from build123d import *

# Parameters (mm, degrees)
EXTRUDE_1_DEPTH          = 4
FILLET_1_R               = 10
SKETCH_2_R               = 7.5
SKETCH_2_R_2             = 1.25
CUT_EXTRUDE_1_DEPTH      = 5
PATTERN_CIRCULAR_1_COUNT = 6
SKETCH_3_R               = 12.5
SKETCH_3_R_2             = 1.25
CUT_EXTRUDE_2_DEPTH      = 5
PATTERN_CIRCULAR_2_COUNT = 4
SKETCH_4_W               = 120
SKETCH_4_H               = 12
CUT_EXTRUDE_3_DEPTH      = 5
FILLET_2_R               = 6
FILLET_3_R               = 6
SKETCH_5_R               = 1.25
CUT_EXTRUDE_5_DEPTH      = 5
PATTERN_LINEAR_2_COUNT   = 3
PATTERN_LINEAR_2_PITCH   = 45


with BuildPart() as part:
    # 草图1 → 凸台-拉伸1 (new body)
    with BuildSketch(Plane.XY):
        with BuildLine():
            Line((18.319446876, 21.832266629), (161.680553124, 21.832266629))
            ThreePointArc((161.680553124, 21.832266629), (208.5, 0), (161.680553124, -21.832266629))
            Line((161.680553124, -21.832266629), (18.319446876, -21.832266629))
            ThreePointArc((18.319446876, -21.832266629), (-28.5, 0), (18.319446876, 21.832266629))
        make_face()
    extrude(amount=EXTRUDE_1_DEPTH)

    # 圆角1
    fillet_1_edges = [part.edges().sort_by_distance(p)[0] for p in [
        (18.319446876, 21.832266629, 2),
        (161.680553124, 21.832266629, 2),
        (161.680553124, -21.832266629, 2),
        (18.319446876, -21.832266629, 2),
    ]]
    fillet(fillet_1_edges, radius=FILLET_1_R)

    # 草图2 → 切除-拉伸1 (cut)
    with BuildSketch(Plane.XY.offset(4)):
        Circle(SKETCH_2_R)
        with Locations((-13.5, 0)):
            Circle(SKETCH_2_R_2)
    cut_extrude_1 = extrude(amount=-CUT_EXTRUDE_1_DEPTH, mode=Mode.SUBTRACT)

    # 阵列(圆周)1: 切除-拉伸1 ×6 about axis
    pattern_circular_1_axis = Axis((0, 0, 0), (0, 0, 1))
    for i in range(1, PATTERN_CIRCULAR_1_COUNT):
        add(cut_extrude_1.rotate(pattern_circular_1_axis, i * 360 / PATTERN_CIRCULAR_1_COUNT), mode=Mode.SUBTRACT)

    # 草图3 → 切除-拉伸2 (cut)
    with BuildSketch(Plane.XY.offset(4)):
        with Locations((180, 0)):
            Circle(SKETCH_3_R)
        with Locations((193.435028843, 13.435028843)):
            Circle(SKETCH_3_R_2)
    cut_extrude_2 = extrude(amount=-CUT_EXTRUDE_2_DEPTH, mode=Mode.SUBTRACT)

    # 阵列(圆周)2: 切除-拉伸2 ×4 about axis
    pattern_circular_2_axis = Axis((180, 0, 0), (0, 0, 1))
    for i in range(1, PATTERN_CIRCULAR_2_COUNT):
        add(cut_extrude_2.rotate(pattern_circular_2_axis, i * 360 / PATTERN_CIRCULAR_2_COUNT), mode=Mode.SUBTRACT)

    # 草图4 → 切除-拉伸3 (cut)
    with BuildSketch(Plane.XY.offset(4)):
        with Locations((90, 0)):
            Rectangle(SKETCH_4_W, SKETCH_4_H)
    extrude(amount=-CUT_EXTRUDE_3_DEPTH, mode=Mode.SUBTRACT)

    # 圆角2
    fillet_2_edges = [part.edges().sort_by_distance(p)[0] for p in [
        (30, 6, 2),
        (30, -6, 2),
    ]]
    fillet(fillet_2_edges, radius=FILLET_2_R - 0.0001)  # a hair under: the kernel refuses the full size

    # 圆角3
    fillet_3_edges = [part.edges().sort_by_distance(p)[0] for p in [
        (150, 6, 2),
        (150, -6, 2),
    ]]
    fillet(fillet_3_edges, radius=FILLET_3_R - 0.0001)  # a hair under: the kernel refuses the full size

    # 草图5 → 切除-拉伸5 (cut)
    with BuildSketch(Plane.XY.offset(4)):
        with Locations((45, 16)):
            Circle(SKETCH_5_R)
        with Locations((45, -16)):
            Circle(SKETCH_5_R)
    cut_extrude_5 = extrude(amount=-CUT_EXTRUDE_5_DEPTH, mode=Mode.SUBTRACT)

    # 阵列(线性)2: 切除-拉伸5 ×3
    with Locations(*[(i * PATTERN_LINEAR_2_PITCH, 0, 0) for i in range(1, PATTERN_LINEAR_2_COUNT)]):
        add(cut_extrude_5, mode=Mode.SUBTRACT)


solid = part.part
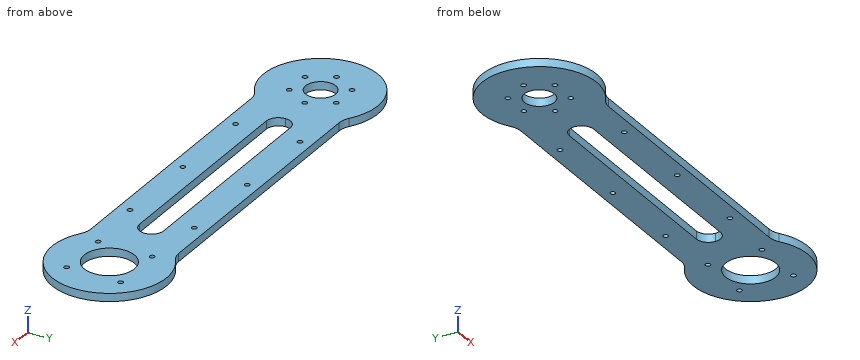
Source: CAD feature listing. Evaluate the final solid. Frame: model axes, mm. Give positions to 0.01 mm unless a question says otherwise; leave off trailing zeros. Write each loop counter-clockwise with the first axis right and the second up, starting at its lowest first coordinate (ties: lowest second). Pieces come first, ordered by that corner, then holes. Notation, with made-up numbers: (1, 20) -> (23, 20) arc R20 cw to (23, 44) -> close; hole circle Ø1 at (72.5, -36.5). An arc over 180 degrees is marked (long way). Return JSON: item names as keys, results as strings. Group by question number.
1. Material intervals for line 1 (Y direction, x = 127, z = 1.45); line 2 (Y direction, x = 91, z = 1.2); line 3 (X direction, y = 17, z = 1.45), sorted ascending. Write a range as from..to.
2. Section C-C, the plane z = 0.85. Count the separate pieces of the cut face and the enclosed holes in it, then the cut area to 3 significant figures.
3. Pin query (flat end, axial travel): pin 1 Ø2 at (x, z) = (91, 2) entering from +Y; pin 2 Ø2 at (x, z) = (123.5, 2.5) entering from -Y. Return the tip coordinate at first contact, or that it passes through.
4. Section A-A, the plane x = 0. Output: boundary loops of the cut face in (y, z), then the cut area to 3 significant figures.
5. Section B-B, the plane x = 180. Output: boundary loops of the cut face in (y, z).
Determined:
{
 "1": {"line 1": "y = -21.83..-6, 6..21.83", "line 2": "y = -21.83..-16.75, -15.25..-6, 6..15.25, 16.75..21.83", "line 3": "x = -22.87..44.25, 45.75..89.25, 90.75..134.25, 135.75..202.87"},
 "2": {"separate pieces": "1", "enclosed holes": "19", "area": "8,590 mm2"},
 "3": {"pin 1": "stops at y = 21.83", "pin 2": "stops at y = -21.83"},
 "4": {"outline": "(-28.5, 0) -> (-7.5, 0) -> (-7.5, 4) -> (-28.5, 4) -> close; (7.5, 0) -> (28.5, 0) -> (28.5, 4) -> (7.5, 4) -> close", "area": "168 mm2"},
 "5": {"outline": "(-28.5, 0) -> (-12.5, 0) -> (-12.5, 4) -> (-28.5, 4) -> close; (12.5, 0) -> (28.5, 0) -> (28.5, 4) -> (12.5, 4) -> close"}
}
